The drawing under review shows one solid part. Ordinate dimensions are in mm from its lowest x, y, z. A direction names the side the tool comes from. Round coordinates to 2 decimals unless told otherwise and drop trailing zeros. Order: outer loops, then holes, each group sorted by start corner. A loop starts at its lowest first (then second) coordinate and runs counter-clockwise, first axis right, second up.
1) Machinability: for the marked faces 1, 2 and 3, which of the approach directions +Z, -Z, +X, -X, +Y, -Y give a long, thin tool a straight path to every point of the face, cutting with its end or side? Answer none if there is none.
2) To check wall thickness, follow L1, parallel to Y at x = 47, z = 90.5. State the ranges of the line that lie inside material, in increasing order.
3) Consider section A-A (z = 84). Give the boundary of the cut face in (x, y), then the cut area to 3 significant figures.
4) Consider section B-B (x = 211). Give the boundary of the cut face in (y, z), then the cut area to 3 significant figures.
5) Clearance check with flat-ended pins moving along their axes: P1, Ø3, axis at y = 1.5, z = 27, coming from the +X side; P2, Ø1.1, axis at y = 3, z = 75.5, coming from the -X side. State where each tip first meets the part, or that it passes through.
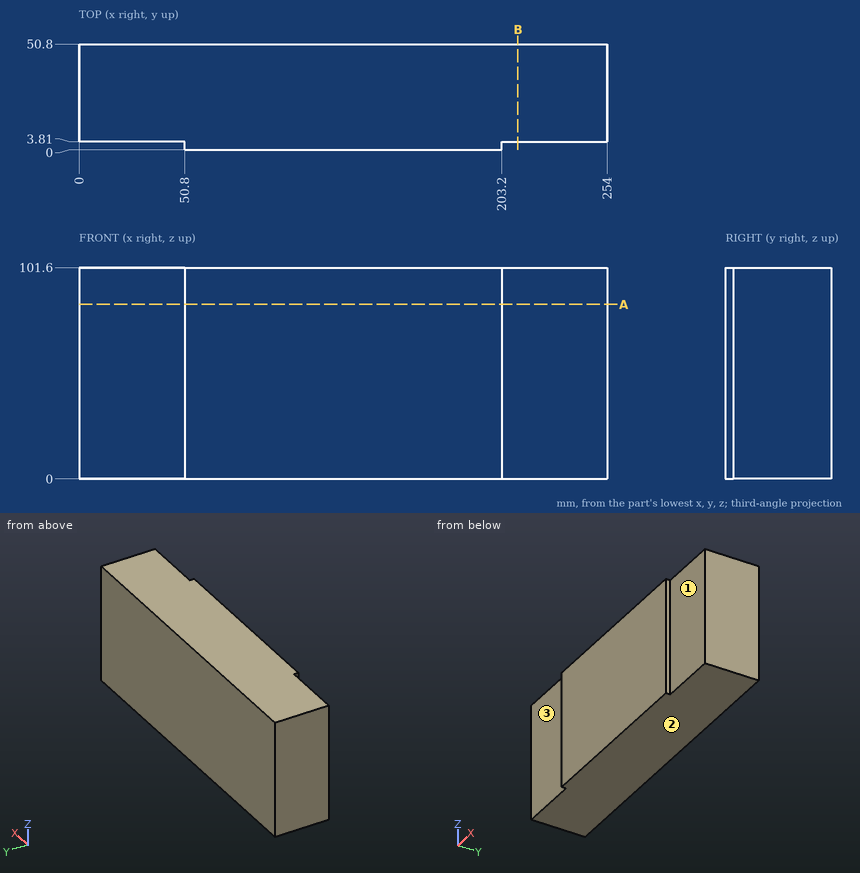
Answer below:
1. face 1: +Z, -Z, +X, -Y
1. face 2: -Z, +X, -X, +Y, -Y
1. face 3: +Z, -Z, -X, -Y
2. L1: y = 3.81 to 50.8
3. outline: (0, 3.81) - (50.8, 3.81) - (50.8, 0) - (203.2, 0) - (203.2, 3.81) - (254, 3.81) - (254, 50.8) - (0, 50.8) - close
3. area: 12,500 mm2
4. outline: (3.81, 0) - (50.8, 0) - (50.8, 101.6) - (3.81, 101.6) - close
4. area: 4,770 mm2
5. P1: stops at x = 203.2
5. P2: stops at x = 50.8
